```python
from build123d import *

# Parameters (mm, degrees)
SKETCH1_R           = 3.175
BOSS_EXTRUDE1_DEPTH = 4.7625


with BuildPart() as part:
    # Sketch1 → Boss-Extrude1 (new body)
    with BuildSketch(Plane.XY):
        Polygon((3.6307971, 110.966804989), (-9.955134074, 19.431), (-4.311994053, 19.431), (-4.311994053, 14.6685), (-10.661994053, 14.6685), (-11.189782837, 11.1125), (-4.311994053, 11.1125), (-4.311994053, 6.35), (-11.896642817, 6.35), (-12.562384724, 1.864534804), (0, 0), (12.7, 85.566804989), (63.5, 85.566804989), (63.5, 110.966804989), align=None)
        with Locations((50.8, 98.266804989)):
            Circle(SKETCH1_R, mode=Mode.SUBTRACT)
    extrude(amount=BOSS_EXTRUDE1_DEPTH)


solid = part.part
```
Model file for the job. Use its own axes, mm. A direction names the side the tool comes from. Give positions to 0.01 mm unless a question says otherwise; leave off trailing zeros. Loops run counter-clockwise (first coordinate to the right, second up) from the corner with the lowest first, then second, coordinate; pieces in that order, holes last. Notation, with made-up numbers: (23.5, 1) - (62.5, 1) arc R36 ccw to (62.5, 39) - close; hole circle Ø3 at (8, 32.25). An arc over 180 degrees is marked (long way). One line per item, written item: value. Start each with the question number.
1. Pull direction Y, two halves, no side cores. Call faces 1 (the flat face through (-12.225, 4.139, 2.348)), 2 (the flat face through (-8, 11.112, 2)), 3 (the flat face through (63.5, 98, 2)): pulls with the +Y half, pulls with the -Y half, needs draft (parallel to the pull), parting line crosses it, or undercut.
2. Pin check, flat tips, straight feed: pin 1 (1.4 mm diameter, centred on x = -9.5, z = 3, fed in from -Y); pin 2 (2.5 mm diameter, centred on y = 16, z = 3.5, fed in from -X). Stop position of each tip, or through.
3. Slice it at C-C (y = 45). List the corners of the cut face in (x, z).
4. Probe L1, parallel to Y at x = 50.8, z = 1.85; L2, parallel to Y at x = 40, z = 4.65; L3, parallel to X at y = 46, z = 3.25. List the from-to ranges inside material, lowest first. Write a range as from..to.
5. Slice it at D-D (x = 8). List the corners of the cut face in (y, z).
6. Slice it at A-A (x = 50.8). List the corners of the cut face in (y, z), plus the area to 3 significant figures.
7. Which spindle directions (+Z, -Z, +X, -X, +Y, -Y) get a long thin tool onto all of the face, cutting with end or side? Do faces 4 (the flat face through (-8, 6.35, 2)), 5 (the flat face through (-3.067, 65.84, 2.348)), 6 (the flat face through (38, 85.567, 2)). Say none if no direction does.
Solution:
1. face 1: pulls with the +Y half
1. face 2: undercut
1. face 3: needs draft
2. pin 1: stops at y = 1.31
2. pin 2: stops at x = -4.31
3. outline: (-6.16, 0) - (6.68, 0) - (6.68, 4.76) - (-6.16, 4.76) - close
4. L1: y = 85.57..95.09, 101.44..110.97
4. L2: y = 85.57..110.97
4. L3: x = -6.01..6.83
5. outline: (53.9, 0) - (110.97, 0) - (110.97, 4.76) - (53.9, 4.76) - close
6. outline: (85.57, 0) - (95.09, 0) - (95.09, 4.76) - (85.57, 4.76) - close; (101.44, 0) - (110.97, 0) - (110.97, 4.76) - (101.44, 4.76) - close
6. area: 90.7 mm^2
7. face 4: +Z, -Z, -X
7. face 5: +Z, -Z, -X, +Y
7. face 6: +Z, -Z, +X, -Y
